```python
from build123d import *

# Parameters (mm, degrees)
SKETCH1_R           = 10
BOSS_EXTRUDE3_DEPTH = 2
CUT_EXTRUDE4_START  = -2
CUT_EXTRUDE4_DEPTH  = 2
CUT_EXTRUDE5_DEPTH  = 2
CUT_EXTRUDE7_START  = -2
CUT_EXTRUDE7_DEPTH  = 2


with BuildPart() as part:
    # Sketch1 → Boss-Extrude3 (new body)
    # profile 1 of 3: a face of its own
    with BuildSketch(Plane(origin=(0, 0, 0), x_dir=(1, 0, 0), z_dir=(0, 1, 0))):
        with BuildLine():
            ThreePointArc((-2.576546391, 9.66237076), (-3.696714803, 9.688501423), (-4.6270391, 10.312966622))
            Line((-4.6270391, 10.312966622), (-5.089759275, 10.867122458))
            add(Edge.make_bspline(
                [(-5.089759275, 10.867122458), (-6.64901802, 12.325915574), (-6.970753087, 12.141194398)],
                knots=[0, 0, 0, 1, 1, 1], degree=2, weights=[1, 1.687053572, 1]))
            ThreePointArc((-6.970753087, 12.141194398), (-7.014608214, -12.115909855), (14, 0))
            ThreePointArc((14, 0), (9.899494937, 9.899494937), (0, 14))
            add(Edge.make_bspline(
                [(-0.996876474, 11.958521535), (-0.370992408, 14), (0, 14)],
                knots=[0, 0, 0, 1, 1, 1], degree=2, weights=[1, 1.687053572, 1]))
            Line((-0.996876474, 11.958521535), (-1.122240194, 11.247548548))
            ThreePointArc((-1.122240194, 11.247548548), (-1.618115564, 10.242776114), (-2.576546391, 9.66237076))
        make_face()
        with BuildLine():
            ThreePointArc((10, 0), (-6.092394278, -7.9298633), (-2.576546391, 9.66237076))
            ThreePointArc((-2.576546391, 9.66237076), (6.092394278, 7.9298633), (10, 0))
        make_face(mode=Mode.SUBTRACT)
    # profile 2 of 3: a face of its own
    with BuildSketch(Plane(origin=(0, 0, 0), x_dir=(1, 0, 0), z_dir=(0, 1, 0))):
        Circle(SKETCH1_R)
    # profile 3 of 3: a face of its own
    with BuildSketch(Plane(origin=(0, 0, 0), x_dir=(1, 0, 0), z_dir=(0, 1, 0))):
        with BuildLine():
            Line((-5.089759275, 10.867122458), (-4.6270391, 10.312966622))
            ThreePointArc((-4.6270391, 10.312966622), (-3.696714803, 9.688501423), (-2.576546391, 9.66237076))
            ThreePointArc((-2.576546391, 9.66237076), (-1.618115564, 10.242776114), (-1.122240194, 11.247548548))
            Line((-1.122240194, 11.247548548), (-0.996876474, 11.958521535))
            add(Edge.make_bspline(
                [(-0.996876474, 11.958521535), (-0.370992408, 14), (0, 14)],
                knots=[0, 0, 0, 1, 1, 1], degree=2, weights=[1, 1.687053572, 1]))
            ThreePointArc((0, 14), (-3.607164983, 13.527319054), (-6.970753087, 12.141194398))
            add(Edge.make_bspline(
                [(-5.089759275, 10.867122458), (-6.64901802, 12.325915574), (-6.970753087, 12.141194398)],
                knots=[0, 0, 0, 1, 1, 1], degree=2, weights=[1, 1.687053572, 1]))
        make_face()
    extrude(amount=BOSS_EXTRUDE3_DEPTH)

    # Sketch2 → Cut-Extrude4 (cut)
    with BuildSketch(Plane(origin=(0, 2, 0), x_dir=(1, 0, 0), z_dir=(0, 1, 0)).offset(CUT_EXTRUDE4_START)):
        with BuildLine():
            Line((-1.136213035, 11.24381356), (-1.010390736, 11.95738728))
            ThreePointArc((-1.010390736, 11.95738728), (-0.613638742, 13.032335811), (0, 14))
            ThreePointArc((0, 14), (-3.623466631, 13.522961568), (-7, 12.124355653))
            ThreePointArc((-7, 12.124355653), (-5.984741166, 11.593153253), (-5.103669595, 10.860596515))
            Line((-5.103669595, 10.860596515), (-4.637917427, 10.305534696))
            ThreePointArc((-4.637917427, 10.305534696), (-2.588190451, 9.659258263), (-1.136213035, 11.24381356))
        make_face()
    extrude(amount=CUT_EXTRUDE4_DEPTH, mode=Mode.SUBTRACT)

    # Sketch3 → Cut-Extrude5 (cut)
    with BuildSketch(Plane(origin=(0, 2, 0), x_dir=(1, 0, 0), z_dir=(0, 1, 0))):
        with BuildLine():
            Line((-2.645751311, 3), (2.645751311, 3))
            ThreePointArc((2.645751311, 3), (4, 0), (2.645751311, -3))
            Line((2.645751311, -3), (-2.645751311, -3))
            ThreePointArc((-2.645751311, -3), (-4, 0), (-2.645751311, 3))
        make_face()
    extrude(amount=-CUT_EXTRUDE5_DEPTH, mode=Mode.SUBTRACT)

    # Sketch2<5> → Cut-Extrude7 (cut)
    with BuildSketch(Plane(origin=(0, 2, 0), x_dir=(1, 0, 0), z_dir=(0, 1, 0)).offset(CUT_EXTRUDE7_START)):
        with BuildLine():
            ThreePointArc((7, 12.124355653), (3.623466631, 13.522961568), (0, 14))
            ThreePointArc((0, 14), (0.613638742, 13.032335811), (1.010390736, 11.95738728))
            Line((1.010390736, 11.95738728), (1.136213035, 11.24381356))
            ThreePointArc((1.136213035, 11.24381356), (2.588190451, 9.659258263), (4.637917427, 10.305534696))
            Line((4.637917427, 10.305534696), (5.103669595, 10.860596515))
            ThreePointArc((5.103669595, 10.860596515), (5.984741166, 11.593153253), (7, 12.124355653))
        make_face()
        with BuildLine():
            ThreePointArc((12.124355653, 7), (9.899494937, 9.899494937), (7, 12.124355653))
            ThreePointArc((7, 12.124355653), (7.047594644, 10.979514512), (6.853717685, 9.850205779))
            Line((6.853717685, 9.850205779), (6.605896133, 9.169321661))
            ThreePointArc((6.605896133, 9.169321661), (7.071067812, 7.071067812), (9.169321661, 6.605896133))
            Line((9.169321661, 6.605896133), (9.850205779, 6.853717685))
            ThreePointArc((9.850205779, 6.853717685), (10.979514512, 7.047594644), (12.124355653, 7))
        make_face()
        with BuildLine():
            ThreePointArc((14, 0), (13.522961568, 3.623466631), (12.124355653, 7))
            ThreePointArc((12.124355653, 7), (11.593153253, 5.984741166), (10.860596515, 5.103669595))
            Line((10.860596515, 5.103669595), (10.305534696, 4.637917427))
            ThreePointArc((10.305534696, 4.637917427), (9.659258263, 2.588190451), (11.24381356, 1.136213035))
            Line((11.24381356, 1.136213035), (11.95738728, 1.010390736))
            ThreePointArc((11.95738728, 1.010390736), (13.032335811, 0.613638742), (14, 0))
        make_face()
        with BuildLine():
            ThreePointArc((-6.853717685, 9.850205779), (-7.047594644, 10.979514512), (-7, 12.124355653))
            ThreePointArc((-7, 12.124355653), (-9.899494937, 9.899494937), (-12.124355653, 7))
            ThreePointArc((-12.124355653, 7), (-10.979514512, 7.047594644), (-9.850205779, 6.853717685))
            Line((-9.850205779, 6.853717685), (-9.169321661, 6.605896133))
            ThreePointArc((-9.169321661, 6.605896133), (-7.071067812, 7.071067812), (-6.605896133, 9.169321661))
            Line((-6.605896133, 9.169321661), (-6.853717685, 9.850205779))
        make_face()
        with BuildLine():
            ThreePointArc((12.124355653, -7), (13.522961568, -3.623466631), (14, 0))
            ThreePointArc((14, 0), (13.032335811, -0.613638742), (11.95738728, -1.010390736))
            Line((11.95738728, -1.010390736), (11.24381356, -1.136213035))
            ThreePointArc((11.24381356, -1.136213035), (9.659258263, -2.588190451), (10.305534696, -4.637917427))
            Line((10.305534696, -4.637917427), (10.860596515, -5.103669595))
            ThreePointArc((10.860596515, -5.103669595), (11.593153253, -5.984741166), (12.124355653, -7))
        make_face()
        with BuildLine():
            ThreePointArc((-10.860596515, 5.103669595), (-11.593153253, 5.984741166), (-12.124355653, 7))
            ThreePointArc((-12.124355653, 7), (-13.522961568, 3.623466631), (-14, 0))
            ThreePointArc((-14, 0), (-13.032335811, 0.613638742), (-11.95738728, 1.010390736))
            Line((-11.95738728, 1.010390736), (-11.24381356, 1.136213035))
            ThreePointArc((-11.24381356, 1.136213035), (-9.659258263, 2.588190451), (-10.305534696, 4.637917427))
            Line((-10.305534696, 4.637917427), (-10.860596515, 5.103669595))
        make_face()
        with BuildLine():
            ThreePointArc((7, -12.124355653), (9.899494937, -9.899494937), (12.124355653, -7))
            ThreePointArc((12.124355653, -7), (10.979514512, -7.047594644), (9.850205779, -6.853717685))
            Line((9.850205779, -6.853717685), (9.169321661, -6.605896133))
            ThreePointArc((9.169321661, -6.605896133), (7.071067812, -7.071067812), (6.605896133, -9.169321661))
            Line((6.605896133, -9.169321661), (6.853717685, -9.850205779))
            ThreePointArc((6.853717685, -9.850205779), (7.047594644, -10.979514512), (7, -12.124355653))
        make_face()
        with BuildLine():
            ThreePointArc((-11.95738728, -1.010390736), (-13.032335811, -0.613638742), (-14, 0))
            ThreePointArc((-14, 0), (-13.522961568, -3.623466631), (-12.124355653, -7))
            ThreePointArc((-12.124355653, -7), (-11.593153253, -5.984741166), (-10.860596515, -5.103669595))
            Line((-10.860596515, -5.103669595), (-10.305534696, -4.637917427))
            ThreePointArc((-10.305534696, -4.637917427), (-9.659258263, -2.588190451), (-11.24381356, -1.136213035))
            Line((-11.24381356, -1.136213035), (-11.95738728, -1.010390736))
        make_face()
        with BuildLine():
            ThreePointArc((0, -14), (3.623466631, -13.522961568), (7, -12.124355653))
            ThreePointArc((7, -12.124355653), (5.984741166, -11.593153253), (5.103669595, -10.860596515))
            Line((5.103669595, -10.860596515), (4.637917427, -10.305534696))
            ThreePointArc((4.637917427, -10.305534696), (2.588190451, -9.659258263), (1.136213035, -11.24381356))
            Line((1.136213035, -11.24381356), (1.010390736, -11.95738728))
            ThreePointArc((1.010390736, -11.95738728), (0.613638742, -13.032335811), (0, -14))
        make_face()
        with BuildLine():
            ThreePointArc((-9.850205779, -6.853717685), (-10.979514512, -7.047594644), (-12.124355653, -7))
            ThreePointArc((-12.124355653, -7), (-9.899494937, -9.899494937), (-7, -12.124355653))
            ThreePointArc((-7, -12.124355653), (-7.047594644, -10.979514512), (-6.853717685, -9.850205779))
            Line((-6.853717685, -9.850205779), (-6.605896133, -9.169321661))
            ThreePointArc((-6.605896133, -9.169321661), (-7.071067812, -7.071067812), (-9.169321661, -6.605896133))
            Line((-9.169321661, -6.605896133), (-9.850205779, -6.853717685))
        make_face()
        with BuildLine():
            ThreePointArc((-7, -12.124355653), (-3.623466631, -13.522961568), (0, -14))
            ThreePointArc((0, -14), (-0.613638742, -13.032335811), (-1.010390736, -11.95738728))
            Line((-1.010390736, -11.95738728), (-1.136213035, -11.24381356))
            ThreePointArc((-1.136213035, -11.24381356), (-2.588190451, -9.659258263), (-4.637917427, -10.305534696))
            Line((-4.637917427, -10.305534696), (-5.103669595, -10.860596515))
            ThreePointArc((-5.103669595, -10.860596515), (-5.984741166, -11.593153253), (-7, -12.124355653))
        make_face()
    extrude(amount=CUT_EXTRUDE7_DEPTH, mode=Mode.SUBTRACT)


solid = part.part
```
Read the model definition and answer for the solid it produces. Units are mm, in the model's axes. A direction names the side the tool comes from. Coordinates: 2 decimals unless noted, no trailing zeros. Order: outer loops, then holes, each group sorted by start corner. A loop starts at its lowest first (then second) coordinate and runs counter-clockwise, first axis right, second up. Notation, with made-up numbers: (11.5, -18.75) - (16.5, -18.75) arc R30 cw to (16.5, 20.25) - close; hole circle Ø10 at (-35.5, 85). An arc over 180 degrees is marked (long way). Answer as a JSON object with one key per item and string values. Group by question number.
Item 1: A tool of negligible diameter and unlimited length cuts with its end or side. For faces 1 (the face through (5.998, 0.986, 11.602)), 2 (the face through (11.602, 0.986, -5.998)), 3 (the face through (-11.602, 0.986, 5.998)), 4 (the face through (0, 1, -3)), from which of +Z, -Z, +X, -X, +Y, -Y can it reach the whole face along a straight path? Write none if from no direction.
Item 2: Section A-A (x = -3) is taken. Give the vertices of the cut face in (y, z), plus the area to 3 significant figures.
Item 3: A flat-ended cylindrical pin translates along its axis: P1, Ø1, axis at x = 8.5, y = 0.5, coming from the +Z side. Find the tip coordinate at first contact, or state that the pin passes through.
Item 4: The mould has two halves that part along X. Classify faces 5 (the face through (13.02, 0.99, -0.62)), 6 (the face through (-11.584, 0.986, -5.971)), 7 (the face through (11, 0.99, 7.05)): +X half, -X half, draft (parallel to the pull), parting line (faces both ways), or undercut.
Item 5: Section C-C (x = 7.75) is taken. Give the vertices of the cut face in (y, z), plus the area to 3 significant figures.
Item 6: Consider probe 1 along Z at (x, y) = (11.5, 1.6); probe 2 along X at (y, z) = (1.35, -10.25). Determine where each line is inside the solid, lowest interval first. Write a range as from..to.
Item 7: Section B-B (z = -3.5) is taken. Give the vertices of the cut face in (x, y).
Results are:
{
 "1": {"face 1": "+Z, +Y, -Y", "face 2": "+X, +Y, -Y", "face 3": "-X, +Y, -Y", "face 4": "+Y, -Y"},
 "2": {"outline": "(0, -9.59) - (2, -9.59) - (2, -2.65) - (0, -2.65) - close; (0, 2.65) - (2, 2.65) - (2, 9.59) - (0, 9.59) - close", "area": "27.8 mm^2"},
 "3": {"P1": "stops at z = 6.55"},
 "4": {"face 5": "+X half", "face 6": "-X half", "face 7": "undercut"},
 "5": {"outline": "(0, -6.63) - (2, -6.63) - (2, 6.63) - (0, 6.63) - close", "area": "26.5 mm^2"},
 "6": {"probe 1": "z = -7.06..-5.85, -1.09..1.09, 5.85..7.06", "probe 2": "x = -6.95..-4.59, -1.62..1.62, 4.59..6.95"},
 "7": {"outline": "(-9.63, 0) - (9.63, 0) - (9.63, 2) - (-9.63, 2) - close"}
}
